from build123d import *

# Parameters (mm, degrees)
SKETCH1_W            = 800
SKETCH1_H            = 450
TABLE_DEPTH          = 50
SKETCH2_W            = 65.292318294
SKETCH2_H            = 35.994240988
PIED_DEPTH           = 500
LPATTERN3_COUNT      = 2
LPATTERN3_PITCH      = 710
LPATTERN3_COUNT_DIR2 = 2
LPATTERN3_PITCH_DIR2 = 360
FILLET1_R            = 10
FILLET2_R            = 10
FILLET3_R            = 10
FILLET4_R            = 10
FILLET5_R            = 10


with BuildPart() as part:
    # Sketch1 → Table (new body)
    with BuildSketch(Plane.XY):
        Rectangle(SKETCH1_W, SKETCH1_H)
    extrude(amount=TABLE_DEPTH)

    # Sketch2 → pied (add)
    with BuildSketch(Plane(origin=(0, 0, 0), x_dir=(-1, 0, 0), z_dir=(0, 0, -1))):
        with Locations((355, -180)):
            Rectangle(SKETCH2_W, SKETCH2_H)
    pied = extrude(amount=PIED_DEPTH)

    # LPattern3: pied 2 × 2
    with Locations(*[(i * LPATTERN3_PITCH, j * LPATTERN3_PITCH_DIR2, 0) for i in range(LPATTERN3_COUNT) for j in range(LPATTERN3_COUNT_DIR2) if (i, j) != (0, 0)]):
        add(pied)

    # Fillet1
    fillet1_edges = [part.edges().sort_by_distance(p)[0] for p in [
        (-400, 0, 50),
        (0, -225, 50),
        (400, 0, 50),
        (0, 225, 50),
    ]]
    fillet(fillet1_edges, radius=FILLET1_R)

    # Fillet2
    fillet2_edges = [part.edges().sort_by_distance(p)[0] for p in [
        (-322.353840853, -162.002879506, -250),
        (-322.353840853, -197.997120494, -250),
        (-387.646159147, -197.997120494, -250),
        (-387.646159147, -162.002879506, -250),
    ]]
    fillet(fillet2_edges, radius=FILLET2_R)

    # Fillet3
    fillet3_edges = [part.edges().sort_by_distance(p)[0] for p in [
        (387.646159147, -162.002879506, -250),
        (387.646159147, -197.997120494, -250),
        (322.353840853, -197.997120494, -250),
        (322.353840853, -162.002879506, -250),
    ]]
    fillet(fillet3_edges, radius=FILLET3_R)

    # Fillet4
    fillet4_edges = [part.edges().sort_by_distance(p)[0] for p in [
        (387.646159147, 162.002879506, -250),
        (387.646159147, 197.997120494, -250),
        (322.353840853, 162.002879506, -250),
        (322.353840853, 197.997120494, -250),
    ]]
    fillet(fillet4_edges, radius=FILLET4_R)

    # Fillet5
    fillet5_edges = [part.edges().sort_by_distance(p)[0] for p in [
        (-322.353840853, 162.002879506, -250),
        (-322.353840853, 197.997120494, -250),
        (-387.646159147, 162.002879506, -250),
        (-387.646159147, 197.997120494, -250),
    ]]
    fillet(fillet5_edges, radius=FILLET5_R)


solid = part.part
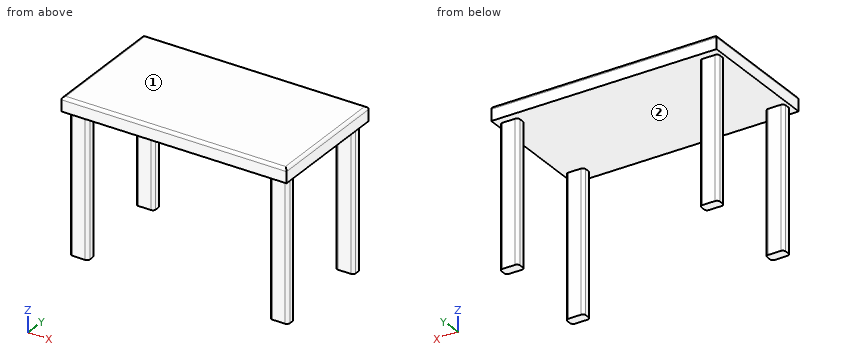
Could you check a few things on this model? Use its own coordinates, in mm. Face numbers are marked on the shaded views. Give positions to 0.01 mm unless a question says otherwise; leave off trailing zeros. Loops run counter-clockwise (first coordinate to the right, second up) from the corner with the lowest first, then second, coordinate; pieces in that order, holes last. Notation, with made-up numbers: (66, 53.25) -> (81, 53.25) arc R11 ccw to (81, 69.25) -> close; hole circle Ø9 at (-34, 45.5). An arc over 180 degrees is marked (long way). Return JSON: item names as keys, results as strings.
Item 1: If we section it at C-C on x = -99: List the corners of the cut face in (y, z) for me, plus the area to 3 significant figures.
Geometry results:
{"outline": "(-225, 0) -> (225, 0) -> (225, 40) arc R10 ccw to (215, 50) -> (-215, 50) arc R10 ccw to (-225, 40) -> close", "area": "22,500 mm²"}
Item 2: If we section it at A-A on z = -353: Count the separate pieces of the cut face and the enclosed holes in it, plus the area to 3 significant figures.
Geometry results:
{"separate pieces": "4", "enclosed holes": "0", "area": "9,060 mm²"}
Item 3: If we section it at B-B on y = 27.5: List the corners of the cut face in (x, z) for me, plus the area to 3 significant figures.
Geometry results:
{"outline": "(-400, 0) -> (400, 0) -> (400, 40) arc R10 ccw to (390, 50) -> (-390, 50) arc R10 ccw to (-400, 40) -> close", "area": "40,000 mm²"}
Item 4: I'm going to push flat-ended pins straight in: pin 1 (2 mm diameter, centred on x = -216.5, y = 35, fed in from -Z); pin 2 (13 mm diameter, centred on y = -182, z = -225, fed in from -X); pin 3 (13.5 mm diameter, centred on x = 362.5, z = -218.5, fed in from +Y). Where does each tip first touch, or does it pass through?
Geometry results:
{"pin 1": "stops at z = 0", "pin 2": "stops at x = -387.65", "pin 3": "stops at y = 198"}
Item 5: We'd pull the mould along Y, two halves only. Please class the marked faces 1 and 2: +Y half, -Y half, draft (parallel to the pull), parting line (faces both ways), or undercut.
Geometry results:
{"face 1": "draft", "face 2": "undercut"}
Item 6: I need wall thicknesses on L1, parallel to Y at x = -363.5, z = -217; L2, parallel to Z at x = -346.5, y = -23; L3, parallel to X at y = 168, z = -15. Which ranges of each line are inside material? Lowest first, please. Write a range as from..to.
Geometry results:
{"L1": "y = -198..-162, 162..198", "L2": "z = 0..50", "L3": "x = -386.81..-323.19, 323.19..386.81"}
